```python
from build123d import *

# Parameters (mm, degrees)
BOSS_EXTRUDE2_DEPTH = 6
SKETCH4_R           = 5
BOSS_EXTRUDE3_DEPTH = 12
SKETCH5_R           = 1.5
CUT_EXTRUDE1_DEPTH  = 6
SKETCH6_R           = 2
CUT_EXTRUDE2_DEPTH  = 12
SKETCH7_R           = 1.5
CUT_EXTRUDE3_DEPTH  = 10


with BuildPart() as part:
    # Sketch3 → Boss-Extrude2 (new body)
    with BuildSketch(Plane.XY):
        Polygon((-4.420907708, 4.056547182), (-5.723526765, -1.800344791), (-1.302619058, -5.856891974), (4.420907708, -4.056547182), (5.723526765, 1.800344791), (1.302619058, 5.856891974), align=None)
    extrude(amount=BOSS_EXTRUDE2_DEPTH)

    # Sketch4 → Boss-Extrude3 (add)
    with BuildSketch(Plane.XY.offset(6)):
        Circle(SKETCH4_R)
    extrude(amount=BOSS_EXTRUDE3_DEPTH)

    # Sketch5 → Cut-Extrude1 (cut, symmetric)
    with BuildSketch(Plane(origin=(0, 0, 0), x_dir=(1, 0, 0), z_dir=(0, 1, 0))):
        with Locations(Location((0, -14.580477712, 0), (0, 0, 270))):
            Circle(SKETCH5_R)
    extrude(amount=CUT_EXTRUDE1_DEPTH, both=True, mode=Mode.SUBTRACT)

    # Sketch6 → Cut-Extrude2 (cut)
    with BuildSketch(Plane.XY.offset(18)):
        Circle(SKETCH6_R)
    extrude(amount=-CUT_EXTRUDE2_DEPTH, mode=Mode.SUBTRACT)

    # Sketch7 → Cut-Extrude3 (cut)
    with BuildSketch(Plane(origin=(0, 0, 0), x_dir=(-1, 0, 0), z_dir=(0, 0, -1))):
        Circle(SKETCH7_R)
    extrude(amount=-CUT_EXTRUDE3_DEPTH, mode=Mode.SUBTRACT)


solid = part.part
```
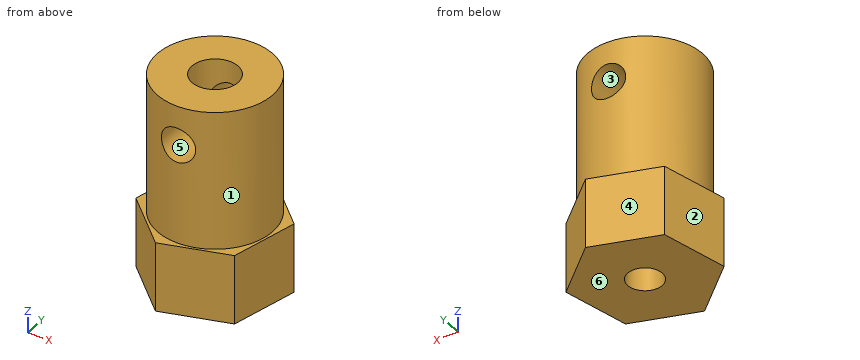
For this review, take the finished solid that the model builds, in its own axes (mm). Face numbers are marked on the shaded views. A direction names the side the tool comes from. Coordinates: 2 decimals unless noted, no trailing zeros. Loops run counter-clockwise (first coordinate to the right, second up) from the corner with the lowest first, then second, coordinate; pieces in that order, holes last. Notation, with made-up numbers: (87.25, -34) - (128.25, -34) arc R13 cw to (128.25, -10) - close; hole circle Ø7 at (4, 7.5). An arc over 180 degrees is marked (long way). Use one line per item in the form item = value. Start each with the question number.
1) To check wall thickness, follow probe 1 along Y at (x, z) = (0, 10); probe 2 along Z at (x, y) = (1.25, 2); probe 3 along Z at (x, y) = (0, 2.9). State the ranges of each line that lie inside material, in increasing order. Write a range as from..to.
2) Take a section at D-D (x = 3). State the section outline as (y, z) points.
3) For the marked faces 1 and 2, list the 3-axis set-ups (+Z, -Z, +X, -X, +Y, -Y) from which the entire face can be reached by the end or side of a thin tool; tool diameter is ignored.
4) Take a section at B-B (x = 0). State the section outline as (y, z) points, plus the area to 3 significant figures.
5) For pin 1 (1.5 mm diameter, centred on x = -3.5, z = 2.5, fed in from -Y); pin 2 (4 mm diameter, centred on x = 2, z = 13, fed in from -Y); pin 3 (4 mm diameter, centred on x = -1, y = -1.5, fed in from +Z); pin 4 (1.8 mm diameter, centred on x = 0, z = 14.58, fed in from -Y), all flat-tipped, find the tip position at first contact; note any pin that passes through.
6) Draft analysis for pull direction Z (two halves, no side actions). For the marked faces 3, 4, 5 and 6, state which applies: released by +Z, released by -Z, zero draft, split by the parting line, or undercut.
7) Take a section at C-C (z = 2). State the section outline as (x, y) points.
8) Take a section at A-A (y = 0). State the section outline as (x, z) points, plus the area to 3 significant figures.
From the geometry:
q1.probe_1 = -5..-2, 2..5
q1.probe_2 = 0..13.75, 15.41..18
q1.probe_3 = 0..13.08, 16.08..18
q2.outline = (-4.5, 0) - (4.3, 0) - (4.3, 6) - (4, 6) - (4, 18) - (-4, 18) - (-4, 6) - (-4.5, 6) - close
q3.face_1 = +Z
q3.face_2 = +Z, -Z, -X, +Y
q4.outline = (-5.45, 0) - (-1.5, 0) - (-1.5, 6) - (-2, 6) - (-2, 13.08) - (-5, 13.08) - (-5, 6) - (-5.45, 6) - close; (-5, 16.08) - (-2, 16.08) - (-2, 18) - (-5, 18) - close; (1.5, 0) - (5.45, 0) - (5.45, 6) - (5, 6) - (5, 13.08) - (2, 13.08) - (2, 6) - (1.5, 6) - close; (2, 16.08) - (5, 16.08) - (5, 18) - (2, 18) - close
q4.area = 101 mm2
q5.pin_1 = -4.53
q5.pin_2 = -5
q5.pin_3 = 18
q5.pin_4 = through
q6.face_3 = undercut
q6.face_4 = zero draft
q6.face_5 = undercut
q6.face_6 = released by -Z
q7.outline = (-5.72, -1.8) - (-1.3, -5.86) - (4.42, -4.06) - (5.72, 1.8) - (1.3, 5.86) - (-4.42, 4.06) - close; hole circle Ø3 at (0, 0)
q8.outline = (-5.32, 0) - (-1.5, 0) - (-1.5, 6) - (-2, 6) - (-2, 18) - (-5, 18) - (-5, 6) - (-5.32, 6) - close; (1.5, 0) - (5.32, 0) - (5.32, 6) - (5, 6) - (5, 18) - (2, 18) - (2, 6) - (1.5, 6) - close
q8.area = 118 mm2
